Work out the finished part from the listing and answer in its coordinate system (mm). Give positions to 0.01 mm unless a question says otherwise; leave off trailing zeros. Write each loop counter-clockwise with the first axis right and the second up, starting at its lowest first coordinate (ties: lowest second). Pieces come first, ordered by that corner, then holes. Notation, with made-up numbers: (-6, 81) -> (23, 81) arc R26 ccw to (23, 100) -> close; hole circle Ø10 at (13.25, 70.25). An arc over 180 degrees is marked (long way). Use a Markdown table: item, result. Add a question column.
Q1. Section A-A, the plane z = 0.7 is taken. Give the vertices of the cut face in (x, y).
Q2. Consider line 1 (X direction, y = 21.5, z = 1.3); line 2 (Y direction, x = -15, z = 1.5); line 3 (X direction, y = -14, z = 0.55). Determine where each line is inside the solid, lowest interval first.
Q3. Section B-B, the plane y = -15 is taken. Give the vertices of the cut face in (x, z), plus the area to 3 significant figures.
Q4. This flat-tipped pin is pushed along its axis until it touches: pin 1 Ø1 at (x, y) = (14.5, -3) entering from -Z. Where does it stop, or does it pass through?
Q5. Section C-C, the plane x = -18 is taken. Give the vertices of the cut face in (y, z).
from build123d import *

# Parameters (mm, degrees)
PAD_DEPTH         = 1.7
POCKET_DEPTH      = 0.001
POCKET_DEPTH_BACK = 1.701


with BuildPart() as part:
    # Sketch001 → Pad (new body)
    with BuildSketch(Plane.XY):
        with BuildLine():
            ThreePointArc((-25.1, -22.029699), (-24.20073, -24.20073), (-22.029699, -25.1))
            Line((22.029699, -25.1), (-22.029699, -25.1))
            ThreePointArc((22.029699, -25.1), (24.20073, -24.20073), (25.1, -22.029699))
            Line((25.1, 22.029699), (25.1, -22.029699))
            ThreePointArc((25.1, 22.029699), (24.20073, 24.20073), (22.029699, 25.1))
            Line((-22.029699, 25.1), (22.029699, 25.1))
            ThreePointArc((-22.029699, 25.1), (-24.20073, 24.20073), (-25.1, 22.029699))
            Line((-25.1, -22.029699), (-25.1, 22.029699))
        make_face()
    extrude(amount=PAD_DEPTH)

    # Binder → Pocket (cut, two sides)
    with BuildSketch(Plane(origin=(-16.970563, -16.970563, 0), x_dir=(0, 1, 0), z_dir=(0, 0, 1))) as pocket_sk:
        with BuildLine():
            ThreePointArc((0.424264, 3.889087), (-3.889087, 3.889087), (-3.889087, -0.424264))
            Line((-3.889087, -0.424264), (-0.424264, -3.889087))
            ThreePointArc((-0.424264, -3.889087), (3.889087, -3.889087), (3.889087, 0.424264))
            Line((3.889087, 0.424264), (0.424264, 3.889087))
        make_face()
        with BuildLine():
            ThreePointArc((-3.889087, -33.516861), (-3.889087, -37.830213), (0.424264, -37.830213))
            Line((0.424264, -37.830213), (3.889087, -34.36539))
            ThreePointArc((3.889087, -34.36539), (3.889087, -30.052038), (-0.424264, -30.052038))
            Line((-0.424264, -30.052038), (-3.889087, -33.516861))
        make_face()
        with BuildLine():
            ThreePointArc((37.830213, -0.424264), (37.830213, 3.889087), (33.516861, 3.889087))
            Line((33.516861, 3.889087), (30.052038, 0.424264))
            ThreePointArc((30.052038, 0.424264), (30.052038, -3.889087), (34.36539, -3.889087))
            Line((34.36539, -3.889087), (37.830213, -0.424264))
        make_face()
        with BuildLine():
            ThreePointArc((33.516861, -37.830213), (37.830213, -37.830213), (37.830213, -33.516861))
            Line((37.830213, -33.516861), (34.36539, -30.052038))
            ThreePointArc((34.36539, -30.052038), (30.052038, -30.052038), (30.052038, -34.36539))
            Line((30.052038, -34.36539), (33.516861, -37.830213))
        make_face()
    extrude(amount=-POCKET_DEPTH, mode=Mode.SUBTRACT)
    extrude(pocket_sk.sketch, amount=POCKET_DEPTH_BACK, mode=Mode.SUBTRACT)


solid = part.part
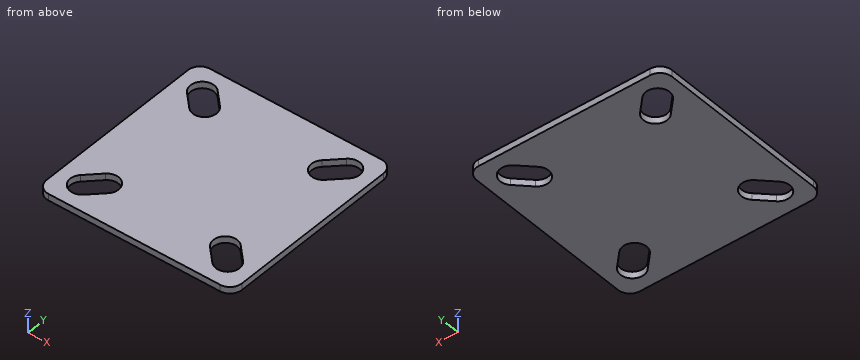
Result set:
| question | item | result |
|---|---|---|
| 1 | outline | (-25.1, -22.03) arc R3.07 ccw to (-22.03, -25.1) -> (22.03, -25.1) arc R3.07 ccw to (25.1, -22.03) -> (25.1, 22.03) arc R3.07 ccw to (22.03, 25.1) -> (-22.03, 25.1) arc R3.07 ccw to (-25.1, 22.03) -> close; hole (-20.86, -16.55) arc R3.05 ccw to (-16.55, -20.86) -> (-13.08, -17.39) arc R3.05 ccw to (-17.39, -13.08) -> close; hole (-20.86, 16.55) -> (-17.39, 13.08) arc R3.05 ccw to (-13.08, 17.39) -> (-16.55, 20.86) arc R3.05 ccw to start; hole (13.08, -17.39) -> (16.55, -20.86) arc R3.05 ccw to (20.86, -16.55) -> (17.39, -13.08) arc R3.05 ccw to start; hole (13.08, 17.39) arc R3.05 ccw to (17.39, 13.08) -> (20.86, 16.55) arc R3.05 ccw to (16.55, 20.86) -> close |
| 2 | line 1 | x = -25.1 to -19.92, -17.49 to 17.49, 19.92 to 25.1 |
| 2 | line 2 | y = -25.1 to -19.31, -12.2 to 12.2, 19.31 to 25.1 |
| 2 | line 3 | x = -25.1 to -18.31, -12.45 to 12.45, 18.31 to 25.1 |
| 3 | outline | (-25.1, 0) -> (-19.31, 0) -> (-19.31, 1.7) -> (-25.1, 1.7) -> close; (-12.2, 0) -> (12.2, 0) -> (12.2, 1.7) -> (-12.2, 1.7) -> close; (19.31, 0) -> (25.1, 0) -> (25.1, 1.7) -> (19.31, 1.7) -> close |
| 3 | area | 61.1 mm2 |
| 4 | pin 1 | stops at z = 0 |
| 5 | outline | (-25.1, 0) -> (-21.67, 0) -> (-21.67, 1.7) -> (-25.1, 1.7) -> close; (-13.69, 0) -> (13.69, 0) -> (13.69, 1.7) -> (-13.69, 1.7) -> close; (21.67, 0) -> (25.1, 0) -> (25.1, 1.7) -> (21.67, 1.7) -> close |
